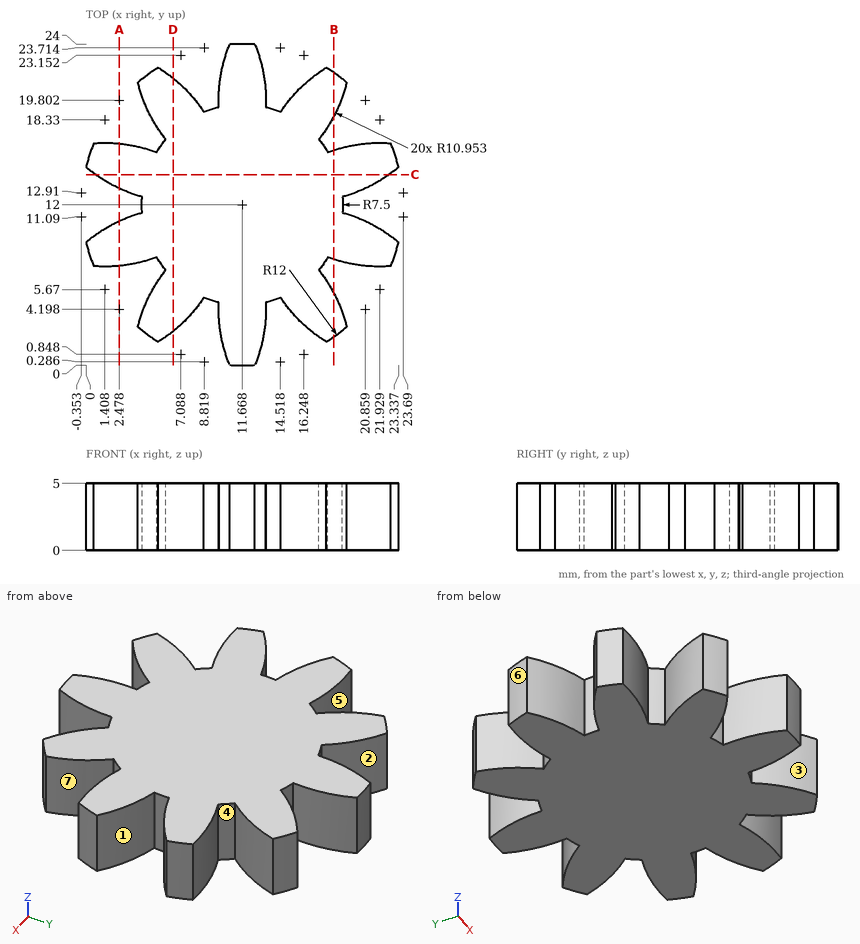
Answer from the drawing. Dimensions are ordinates in mm from the lowest x, y and z of the part. A direction names the side the tool comes from. Coordinates: 2 decimals unless noted, no trailing zeros. Write each loop counter-clockwise with the first axis right and the second up, starting at its lowest first coordinate (ties: lowest second). Pieces come first, ordered by that corner, then holes. Notation, with made-up numbers: M 23.5,-13.75 L 79.5,-13.75 A25 cw 79.5,24.25 Z; hole C 60.25,61 d3. An arc over 180 degrees is marked long. Use a Markdown table: item, result.
Q1. The part is cut by section D-D, the plane x = 6.5. Write down the section's boundary in (y, z) (1 decimal).
Answer block:
| item | result |
|---|---|
| outline | M 2.5,0 L 21.5,0 L 21.5,5 L 2.5,5 Z |
Q2. The part is cut by section C-C, the plane y = 14.25. Write down the section's boundary in (x, z), then the cut area to 3 significant figures.
Answer block:
| item | result |
|---|---|
| outline | M 0.71,0 L 22.63,0 L 22.63,5 L 0.71,5 Z |
| area | 110 mm2 |
Q3. The part is cut by section B-B, the plane x = 18.5. Write down the section's boundary in (y, z) (1 decimal).
Answer block:
| item | result |
|---|---|
| outline | M 2.1,0 L 5.4,0 L 5.4,5 L 2.1,5 Z; M 7.9,0 L 16.1,0 L 16.1,5 L 7.9,5 Z; M 18.6,0 L 21.9,0 L 21.9,5 L 18.6,5 Z |
Q4. The part is cut by section A-A, the plane x = 2.5. Write down the section's boundary in (y, z) (1 decimal).
Answer block:
| item | result |
|---|---|
| outline | M 7.4,0 L 10.8,0 L 10.8,5 L 7.4,5 Z; M 13.2,0 L 16.6,0 L 16.6,5 L 13.2,5 Z |
Q5. Determine the mould class of the marked faces 5, 6 and 7 for opening direction X: released by +X, released by -X, zero draft, split by the parting line, or undercut.
Answer block:
| item | result |
|---|---|
| face 5 | undercut |
| face 6 | released by -X |
| face 7 | released by +X |
Q6. Which of the six approach directions +Z, -Z, +X, -X, +Y, -Y give full straight-line access (tool end or side, diameter ignored) to the marked faces 1, 2, 3 and 4?
Answer block:
| item | result |
|---|---|
| face 1 | +Z, -Z, +X |
| face 2 | +Z, -Z, +Y |
| face 3 | +Z, -Z, -Y |
| face 4 | +Z, -Z |
Q7. Straight lines are drawn through the part: L1, parallel to X at y = 2, z = 0.5 (1 decimal); L2, parallel to X at y = 20.75, z = 1.5 (1 decimal); L3, parallel to Y at x = 1, z = 1.05 (1 decimal). For each, find the intervals that lie inside material, in ascending order. Write a range as [from, to].
Answer block:
| item | result |
|---|---|
| L1 | x = [5, 5.8], [10.1, 13.2], [17.6, 18.3] |
| L2 | x = [4, 7.3], [9.9, 13.4], [16, 19.4] |
| L3 | y = [7.4, 10], [14, 16.6] |
Q8. Each of these flat-tipped pins is pushed along its axis until it touches: pin 1 Ø2 at (x, z) = (10.5, 1) entering from -Y; pin 2 Ø1.5 at (x, z) = (15, 2) entering from +Y (1 decimal). Where does it stop, or does it pass through?
Answer block:
| item | result |
|---|---|
| pin 1 | stops at y = 0 |
| pin 2 | stops at y = 20.5 |
